from build123d import *

# Parameters (mm, degrees)
BOSS_EXTRUDE1_DEPTH = 5.08
BOSS_EXTRUDE2_DEPTH = 57.15
BOSS_EXTRUDE3_DEPTH = 63.5
BOSS_EXTRUDE4_DEPTH = 63.5
BOSS_EXTRUDE5_DEPTH = 57.15
SKETCH7_W           = 292.1
SKETCH7_H           = 304.8
BOSS_EXTRUDE6_DEPTH = 2.54


with BuildPart() as part:
    # Sketch1 → Boss-Extrude1 (new body)
    with BuildSketch(Plane.XY):
        with BuildLine():
            Line((-88.9, 152.4), (-88.9, 12.7))
            ThreePointArc((-88.9, 12.7), (0, -76.2), (88.9, 12.7))
            Line((88.9, 12.7), (88.9, 152.4))
            Line((88.9, 152.4), (146.05, 152.4))
            Line((146.05, 152.4), (146.05, -152.4))
            Line((146.05, -152.4), (-146.05, -152.4))
            Line((-146.05, -152.4), (-146.05, 152.4))
            Line((-146.05, 152.4), (-88.9, 152.4))
        make_face()
    extrude(amount=BOSS_EXTRUDE1_DEPTH)

    # Sketch2 → Boss-Extrude2 (add)
    with BuildSketch(Plane(origin=(146.05, 0, 0), x_dir=(0, 0, -1), z_dir=(1, 0, 0))):
        Polygon((-5.08, 152.4), (-243.014423739, 342.9), (-237.934423739, 342.9), (0, 152.4), align=None)
    extrude(amount=-BOSS_EXTRUDE2_DEPTH)

    # Sketch3 → Boss-Extrude3 (add)
    with BuildSketch(Plane(origin=(0, 0, 0), x_dir=(-1, 0, 0), z_dir=(0, 0, -1))):
        Polygon((141.934676661, -147.172428926), (-142.059608363, -147.172428926), (-142.059608363, 152.4), (-146.05, 152.4), (-146.05, -152.4), (146.05, -152.4), (146.05, 152.4), (141.934676661, 152.4), align=None)
    extrude(amount=BOSS_EXTRUDE3_DEPTH)

    # Sketch4 → Boss-Extrude4 (add)
    with BuildSketch(Plane(origin=(0, 0, -63.5), x_dir=(-1, 0, 0), z_dir=(0, 0, -1))):
        Polygon((-146.05, 152.4), (-214.625070232, 309.862442089), (-210.634678595, 309.862442089), (-142.059608363, 152.4), align=None)
    boss_extrude4 = extrude(amount=-BOSS_EXTRUDE4_DEPTH)

    # Mirror3: Boss-Extrude4 across plane
    add(boss_extrude4.mirror(Plane(origin=(0, 0, 0), x_dir=(0, 0, 1), z_dir=(1, 0, 0))))

    # Sketch6 → Boss-Extrude5 (add)
    with BuildSketch(Plane(origin=(-88.9, 0, 0), x_dir=(0, 0, -1), z_dir=(1, 0, 0))):
        Polygon((-5.08, 152.4), (-243.014423739, 342.9), (-237.934423739, 342.9), (0, 152.4), align=None)
    extrude(amount=-BOSS_EXTRUDE5_DEPTH)

    # Sketch7 → Boss-Extrude6 (add)
    with BuildSketch(Plane(origin=(0, 0, -63.5), x_dir=(-1, 0, 0), z_dir=(0, 0, -1))):
        Rectangle(SKETCH7_W, SKETCH7_H)
    extrude(amount=BOSS_EXTRUDE6_DEPTH)


solid = part.part
Input: part model. Units: mm. Frame: model coordinates. A direction names the side the tool comes from. Give positions to 0.01 mm unless a question says otherwise; leave off trailing zeros. Write each loop counter-clockwise with the first axis right and the second up, starting at its lowest first coordinate (ties: lowest second). Pieces come first, ordered by that corner, then holes. Notation, with made-up numbers: (61.5, -25) -> (74.5, -25) arc R31 ccw to (74.5, 11) -> close; hole circle Ø6 at (31.5, 68). An arc over 180 degrees is marked (long way). Use one line per item in the form item = value. Start each with the question number.
1) Set-up query: faces 1 (the flat face through (2, -99, 5.08)), 2 (the flat face through (2, 5, -63.5)), 3 (the flat face through (2, -152.4, -30)), 4 (the flat face through (-88.9, 166.3, 21.9)). Return all of +Z, -Z, +X, -X, +Y, -Y with unobstructed straight access to the full face (end or side cutting, diameter ignored); none if empty.
2) Section query A-A on y = -97. Return the cut outline in (x, z), then the cut area to 3 significant figures.
3) Pin query (flat end, axial travel): pin 1 (12 mm diameter, centred on x = 166.5, y = 236.5, fed in from -Z); pin 2 (5 mm diameter, centred on y = 136, z = -20, fed in from +X); pin 3 (1.2 mm diameter, centred on x = 212.5, z = -18.5, fed in from +Y); pin 4 (3 mm diameter, centred on x = 99, y = -40.5, fed in from +Z). Return the tip coordinate at first contact, or that it passes through.
4) Section query C-C on z = -14. Return the cut outline in (x, y).
5) Ray query, probe 1 along X at (y, z) = (110, -47); probe 2 along Z at (x, y) = (-42, 75); probe 3 along Z at (x, y) = (-114, -118). Return the intervals inside material, ascending. Write a range as from..to.
6) Section query D-D on y = 85.5. Return the cut outline in (x, z).
7) Section query B-B on x = -130.5. Return the cut outline in (y, z), then the cut area to 3 significant figures.
8) Draft query along Z for faces 5 (the flat face through (117.875, 246.317, 122.382)), 6 (the flat face through (179.86, 230.03, -32.19)), 7 (the flat face through (-141.935, 5, -31)). Return one class per face: pulls with the +Z half, pulls with the -Z half, needs draft (parallel to the pull), parting line crosses it, or undercut.
Outcome:
q1.face_1 = +Z, +X, -X, -Y
q1.face_2 = +Y
q1.face_3 = +Z, -Z, +X, -X, -Y
q1.face_4 = +Z, +Y
q2.outline = (-146.05, -66.04) -> (146.05, -66.04) -> (146.05, 5.08) -> (-146.05, 5.08) -> close; hole (-141.93, -63.5) -> (142.06, -63.5) -> (142.06, 0) -> (-141.93, 0) -> close
q2.area = 2,740 mm^2
q3.pin_1 = through
q3.pin_2 = 146.05
q3.pin_3 = 309.86
q3.pin_4 = 5.08
q4.outline = (-214.63, 309.86) -> (-146.05, 152.4) -> (-146.05, -152.4) -> (146.05, -152.4) -> (146.05, 152.4) -> (214.63, 309.86) -> (210.63, 309.86) -> (142.06, 152.4) -> (142.06, -147.17) -> (-141.93, -147.17) -> (-141.93, 152.4) -> (-142.06, 152.4) -> (-210.63, 309.86) -> close
q5.probe_1 = -146.05..-141.93, 142.06..146.05
q5.probe_2 = -66.04..-63.5
q5.probe_3 = -66.04..-63.5, 0..5.08
q6.outline = (-146.05, -66.04) -> (146.05, -66.04) -> (146.05, 5.08) -> (88.9, 5.08) -> (88.9, 0) -> (142.06, 0) -> (142.06, -63.5) -> (-141.93, -63.5) -> (-141.93, 0) -> (-88.9, 0) -> (-88.9, 5.08) -> (-146.05, 5.08) -> close
q7.outline = (-152.4, -66.04) -> (152.4, -66.04) -> (152.4, -63.5) -> (-147.17, -63.5) -> (-147.17, 0) -> (152.4, 0) -> (342.9, 237.93) -> (342.9, 243.01) -> (152.4, 5.08) -> (-152.4, 5.08) -> close
q7.area = 3,620 mm^2
q8.face_5 = pulls with the +Z half
q8.face_6 = needs draft
q8.face_7 = undercut
